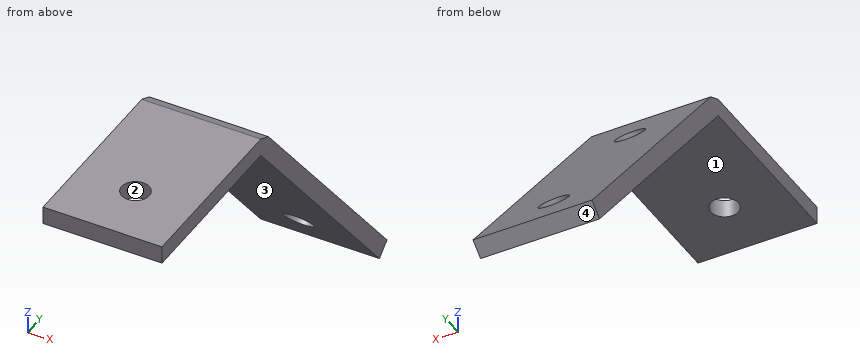
```python
from build123d import *

# Parameters (mm, degrees)
SKETCH_2_W          = 3
SKETCH_2_H          = 30
EXTRUDE_1_DEPTH     = 20
CUT_EXTRUDE_1_REACH = 83.569
SKETCH_3_R          = 2.5
SKETCH_4_R          = 2.328749205
CUT_EXTRUDE_2_DEPTH = 100


with BuildPart() as part:
    # Sketch 2 → Extrude 1 (new body)
    with BuildSketch(Plane(origin=(0, 0, 0), x_dir=(0, 0, -1), z_dir=(1, 0, 0))):
        Polygon((3, 30), (45.898488815, 65.996106142), (43.970125986, 68.294239472), (1.071637171, 32.298133329), align=None)
        Polygon((3, 30), (1.071637171, 32.298133329), (0, 30), align=None)
        with Locations((1.5, 15)):
            Rectangle(SKETCH_2_W, SKETCH_2_H)
    extrude(amount=EXTRUDE_1_DEPTH)

    # Sketch 3 → Cut-Extrude 1 (cut, up to next)
    with BuildSketch(Plane(origin=(0, 16.127511035, 13.532588562), x_dir=(-1, 0, 0), z_dir=(0, -0.7660444431189622, -0.6427876096865582)), mode=Mode.PRIVATE) as cut_extrude_1_sk1:
        with Locations(Location((-10, 67.58176162, 0), (0, 0, 90))):
            Circle(SKETCH_3_R)
    cut_extrude_1_tool1 = extrude(cut_extrude_1_sk1.sketch, amount=-CUT_EXTRUDE_1_REACH, mode=Mode.PRIVATE) & part.part
    # Sketch 3 → Cut-Extrude 1 (cut, up to next)
    with BuildSketch(Plane(origin=(0, 16.127511035, 13.532588562), x_dir=(-1, 0, 0), z_dir=(0, -0.7660444431189622, -0.6427876096865582)), mode=Mode.PRIVATE) as cut_extrude_1_sk2:
        with Locations(Location((-10, 31.58176162, 0), (0, 0, 90))):
            Circle(SKETCH_3_R)
    cut_extrude_1_tool2 = extrude(cut_extrude_1_sk2.sketch, amount=-CUT_EXTRUDE_1_REACH, mode=Mode.PRIVATE) & part.part
    add(cut_extrude_1_tool1.solids().sort_by_distance((10, 59.56823, -38.238044))[0], mode=Mode.SUBTRACT)
    add(cut_extrude_1_tool2.solids().sort_by_distance((10, 36.427876, -10.660444))[0], mode=Mode.SUBTRACT)

    # Sketch 4 → Cut-Extrude 2 (cut)
    with BuildSketch(Plane(origin=(0, 0, -3), x_dir=(-1, 0, 0), z_dir=(0, 0, -1))):
        with Locations((-10, 10)):
            Circle(SKETCH_4_R)
    extrude(amount=-CUT_EXTRUDE_2_DEPTH, mode=Mode.SUBTRACT)


solid = part.part
```
Verification items for the finished model (mm, model axes). Face numbers are marked on the shaded views. Coordinates: 2 decimals unless noted, no trailing zeros. Write each loop counter-clockwise with the first axis right and the second up, starting at its lowest first coordinate (ties: lowest second). Pieces come first, ordered by that corner, then holes. Notation, with made-up numbers: M 39,-25 L 94,-25 A11 ccw 94,-10 Z; hole C -2.5,2.25 d7. An arc over 180 degrees is marked long. Answer as a JSON object with one key per item and string values. Group by question number.
(1) Cross-section at D-D, the plane y = 19. Record the cut outline in (x, z), and give its area (3 significant figures).
(2) Gauge pin test, flat ends, axial feed: pin 1 (6 mm diameter, centred on x = 14.5, y = 44, fed in from +Z); pin 2 (5 mm diameter, centred on x = 7.5, y = 40, fed in from +Z); pin 3 (4 mm diameter, centred on x = 3.5, z = -5.5, fed in from +Y). Record the tip position at first contact, or that the pin passes through.
(3) Release check for a two-part mould opening along Y. For the marked faces 1, 2, 3 and 4 record: +Y half, -Y half, draft (parallel to the pull), parting line (faces both ways), or undercut.
(4) Cross-section at A-A, the plane y = 10. Record the cut outline in (x, z).
(5) Material ranges on line 1 (Z direction, x = 17.5, y = 18); line 2 (Y direction, x = 10, z = -1.85); line 3 (Y direction, x = 10, z = -1.6), recorded low to high.
(6) Cross-section at C-C, the plane x = 2.5. Record the cut outline in (y, z).
(7) Cross-section at B-B, the plane x = 10. Record the cut outline in (y, z), and give its area (3 significant figures).
Reply:
{
 "1": {"outline": "M 0,-3 L 20,-3 L 20,0 L 0,0 Z", "area": "60.0 mm²"},
 "2": {"pin 1": "z = -11.44", "pin 2": "z = -7.27", "pin 3": "y = 37.69"},
 "3": {"face 1": "draft", "face 2": "undercut", "face 3": "-Y half", "face 4": "+Y half"},
 "4": {"outline": "M 0,-3 L 7.67,-3 L 7.67,0 L 0,0 Z; M 12.33,-3 L 20,-3 L 20,0 L 12.33,0 Z"},
 "5": {"line 1": "-3 to 0", "line 2": "0 to 7.67, 12.33 to 32.95", "line 3": "0 to 7.67, 12.33 to 32.74"},
 "6": {"outline": "M 0,-3 L 30,-3 L 66,-45.9 L 68.29,-43.97 L 32.3,-1.07 L 30,0 L 0,0 Z"},
 "7": {"outline": "M 0,-3 L 7.67,-3 L 7.67,0 L 0,0 Z; M 12.33,-3 L 30,-3 L 34.82,-8.75 L 37.12,-6.82 L 32.3,-1.07 L 30,0 L 12.33,0 Z; M 38.03,-12.58 L 57.96,-36.32 L 60.26,-34.39 L 40.33,-10.65 Z; M 61.18,-40.15 L 66,-45.9 L 68.29,-43.97 L 63.47,-38.22 Z", "area": "217 mm²"}
}
